```python
from build123d import *

# Parameters (mm, degrees)
BOSS_EXTRUDE1_DEPTH = 43.2
DRAFT2_ANGLE        = 8


with BuildPart() as part:
    # Sketch3 → Boss-Extrude1 (new body)
    with BuildSketch(Plane(origin=(0, 24, 0), x_dir=(1, 0, 0), z_dir=(0, 1, 0))):
        with BuildLine():
            Line((-0.896175087, -52.835898714), (0.896175087, -52.835898714))
            ThreePointArc((0.896175087, -52.835898714), (24.408925383, -48.242362776), (46.481310912, -38.927868909))
            ThreePointArc((46.481310912, -38.927868909), (67.768695813, -34.318589585), (89.02611517, -39.064148992))
            Line((89.02611517, -39.064148992), (120, -39.064148992))
            Line((120, -39.064148992), (120, -30))
            Line((120, -30), (93.25, -30))
            ThreePointArc((93.25, -30), (67.606257623, -24.318329423), (41.962515246, -30))
            ThreePointArc((41.962515246, -30), (21.653208784, -38.627914511), (0, -42.876136156))
            ThreePointArc((0, -42.876136156), (-21.653208784, -38.627914511), (-41.962515246, -30))
            ThreePointArc((-41.962515246, -30), (-67.606257623, -24.318329423), (-93.25, -30))
            Line((-93.25, -30), (-110, -30))
            Line((-110, -30), (-110, -39.064148992))
            Line((-110, -39.064148992), (-89.02611517, -39.064148992))
            ThreePointArc((-89.02611517, -39.064148992), (-67.768695813, -34.318589585), (-46.481310912, -38.927868909))
            ThreePointArc((-46.481310912, -38.927868909), (-24.408925383, -48.242362776), (-0.896175087, -52.835898714))
        make_face()
    extrude(amount=-BOSS_EXTRUDE1_DEPTH)

    # Draft2
    draft2_faces = [part.faces().sort_by_distance(p)[0] for p in [
        (0, 2.4, 52.835898714),
        (104.513057585, 2.4, 39.064148992),
        (67.768695813, 2.4, 34.318589585),
        (24.408925383, 2.4, 48.242362776),
        (-24.408925383, 2.4, 48.242362776),
        (-67.768695813, 2.4, 34.318589585),
        (-99.513057585, 2.4, 39.064148992),
    ]]
    draft(draft2_faces, Plane.ZX.offset(24), DRAFT2_ANGLE)


solid = part.part
```
CAD build for the part. Positions are in the model's coordinates, mm. A direction names the side the tool comes from. Give positions to 0.01 mm unless a question says otherwise; leave off trailing zeros. Order: outer loops, then holes, each group sorted by start corner. A loop starts at its lowest first (then second) coordinate and runs counter-clockwise, first axis right, second up.
(1) Saw through at A-A, the plane y = 18.5. Give the cut face in (x, z).
(2) Mould opens along X. For faces 1 (the flat face through (-110, 3, 36)), 2 (the flat face through (-102, 3, 30)), 3 (the conical face through (68.157, 2.702, 37.315)) say: released by +X, released by -X, zero draft, split by the parting line, or undercut.
(3) Flat gauge pins, fed straight in: pin 1 (12 mm diameter, centred on x = -3, y = 1, fed in from +Z); pin 2 (10 mm diameter, centred on y = 14, z = 43, fed in from -X); pin 3 (12 mm diameter, centred on x = 63.5, y = 13, fed in from +Z); pin 4 (8 mm diameter, centred on x = 103.5, y = -7, fed in from -Z). Where does each tip first touch, or does it go through?
(4) Tool access for faces 4 (the flat face through (-98.974, 2.702, 42.057)), 5 (the flat face through (103.591, 2.702, 42.057)), 6 (the flat face through (-0.02, 2.7, 55.83)), 7 (the flat face through (107, 3, 30)), 8 (the cylindrical face through (-21.357, 2.702, 38.718)): list every direction of +Z, -Z, +X, -X, +Y, -Y with a clear straight run to the whole face (end or side of a thin tool).
(5) Saw through at B-B, the plane y = 3.5. Give the cut face in (x, z) (3 decimals).
(6) Drill centre lines: L1, parallel to X at y = 11, z = 30.5; L2, parallel to X at y = 14.5, z = 34; L3, parallel to Z at x = 35, y = 7. Where is each one in solid material? Low to high.
Results found:
1. outline: (-110, 30) - (-93.25, 30) arc R60.71 ccw to (-41.96, 30) arc R106.28 cw to (0, 42.88) arc R106.28 cw to (41.96, 30) arc R60.71 ccw to (93.25, 30) - (120, 30) - (120, 39.84) - (88.85, 39.84) arc R49.94 cw to (46.83, 39.62) arc R117.06 ccw to (0.93, 53.61) - (-0.93, 53.61) arc R117.06 ccw to (-46.83, 39.62) arc R49.94 cw to (-88.85, 39.84) - (-110, 39.84) - close
2. face 1: released by -X
2. face 2: zero draft
2. face 3: undercut
3. pin 1: stops at z = 56.87
3. pin 2: stops at x = -110
3. pin 3: stops at z = 37.19
3. pin 4: stops at z = 30
4. face 4: +Z, -X, +Y
4. face 5: +Z, +X, +Y
4. face 6: +Z, +X, -X, +Y
4. face 7: -Z, +X, +Y, -Y
4. face 8: -Z, +Y, -Y
5. outline: (-110, 30) - (-93.25, 30) arc R60.711 ccw to (-41.963, 30) arc R106.283 cw to (0, 42.876) arc R106.283 cw to (41.963, 30) arc R60.711 ccw to (93.25, 30) - (120, 30) - (120, 41.945) - (88.378, 41.945) arc R47.83 cw to (47.775, 41.504) arc R119.164 ccw to (1.025, 55.717) - (-1.025, 55.717) arc R119.164 ccw to (-47.775, 41.504) arc R47.83 cw to (-88.378, 41.945) - (-110, 41.945) - close
6. L1: x = -110 to -41.05, 41.05 to 120
6. L2: x = -110 to -33.96, 33.96 to 120
6. L3: z = 33.53 to 47.02
